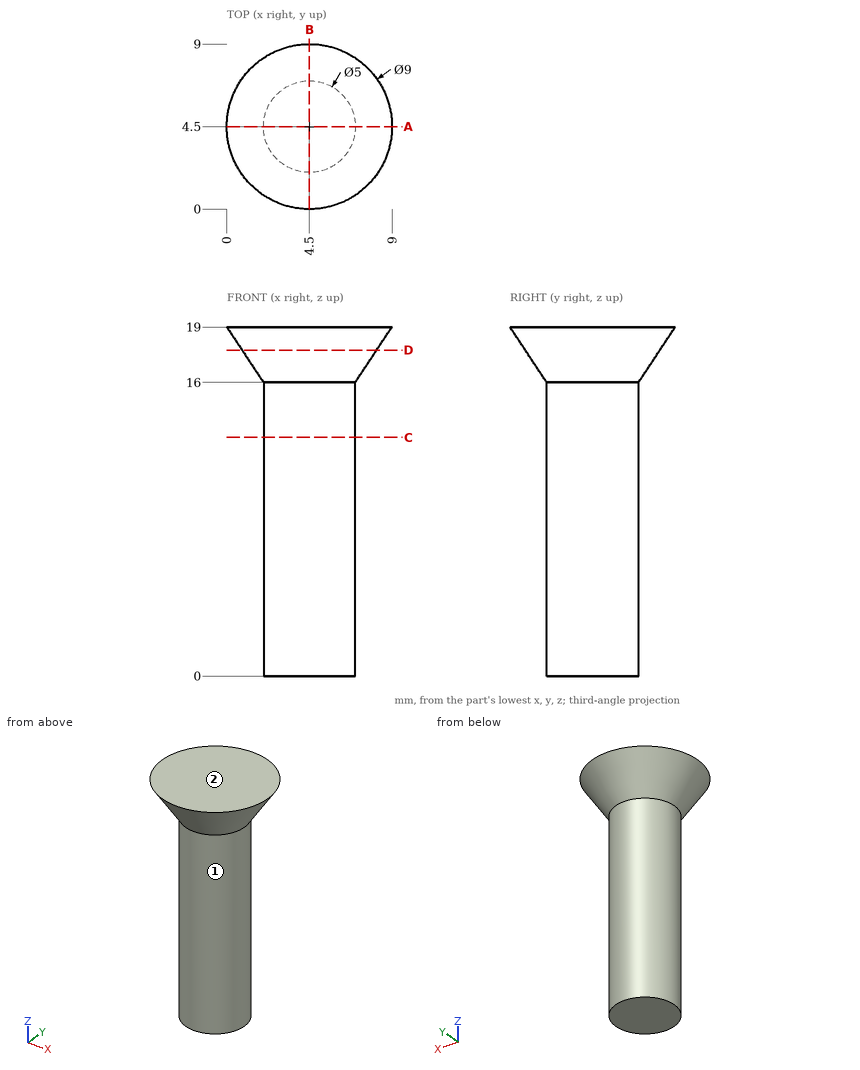
Here's the drawing with two shaded views (mm, measured from the low corner). I have some questions. A direction names the side the tool comes from. Coordinates: 2 decimals unless noted, no trailing zeros. Write each loop counter-clockwise with the first axis right and the second up, starting at its lowest first coordinate (ties: lowest second). Pieces come first, ordered by that corner, then holes. Notation, with made-up numbers: (-14.75, 59) -> (24.25, 59) arc R23 ccw to (24.25, 83) -> close; hole circle Ø8 at (-27.75, 49.25). An arc over 180 degrees is marked (long way). Write item = value, one per line. Start each with the question number.
(1) I want a section at D-D (z = 17.75). Please give me the cut outline in (x, y).
(2) Which directions (+Z, -Z, +X, -X, +Y, -Y) give clear straight access to the entire face, cutting with the end or side of a thin tool? Please do the marked faces 1 and 2.
(3) Will these pins go through, and if not, where does the flat tip stop? pin 1 (4 mm diameter, centred on x = 7.5, z = 16, fed in from +Y); pin 2 (1.5 mm diameter, centred on y = 7, z = 8.5, fed in from -X); pin 3 (4 mm diameter, centred on y = 6, z = 12, fed in from -X); pin 4 (3 mm diameter, centred on x = 7, y = 7.5, fed in from -Z).
(4) I want a section at A-A (y = 4.5). Please give me the cut outline in (x, z), plus the area to 3 significant figures.
(5) I need wall thicknesses on line 1 (Z direction, x = 8.5, y = 3.5); line 2 (Y direction, x = 3.25, z = 15.5); line 3 (Y direction, x = 4.5, z = 8.25). Which ranges of each line are inside material? Lowest first, please. Write a range as [from, to].
(6) I want a section at C-C (z = 13). Please give me the cut outline in (x, y), plus the area to 3 significant figures.
Result set:
q1.outline = circle Ø7.33 at (4.5, 4.5)
q2.face_1 = -Z
q2.face_2 = +Z, +X, -X, +Y, -Y
q3.pin_1 = 7.58
q3.pin_2 = 2.71
q3.pin_3 = 2
q3.pin_4 = 0
q4.outline = (0, 19) -> (2, 16) -> (2, 0) -> (7, 0) -> (7, 16) -> (9, 19) -> close
q4.area = 101 mm2
q5.line_1 = [18.43, 19]
q5.line_2 = [2.33, 6.67]
q5.line_3 = [2, 7]
q6.outline = circle Ø5 at (4.5, 4.5)
q6.area = 19.6 mm2
